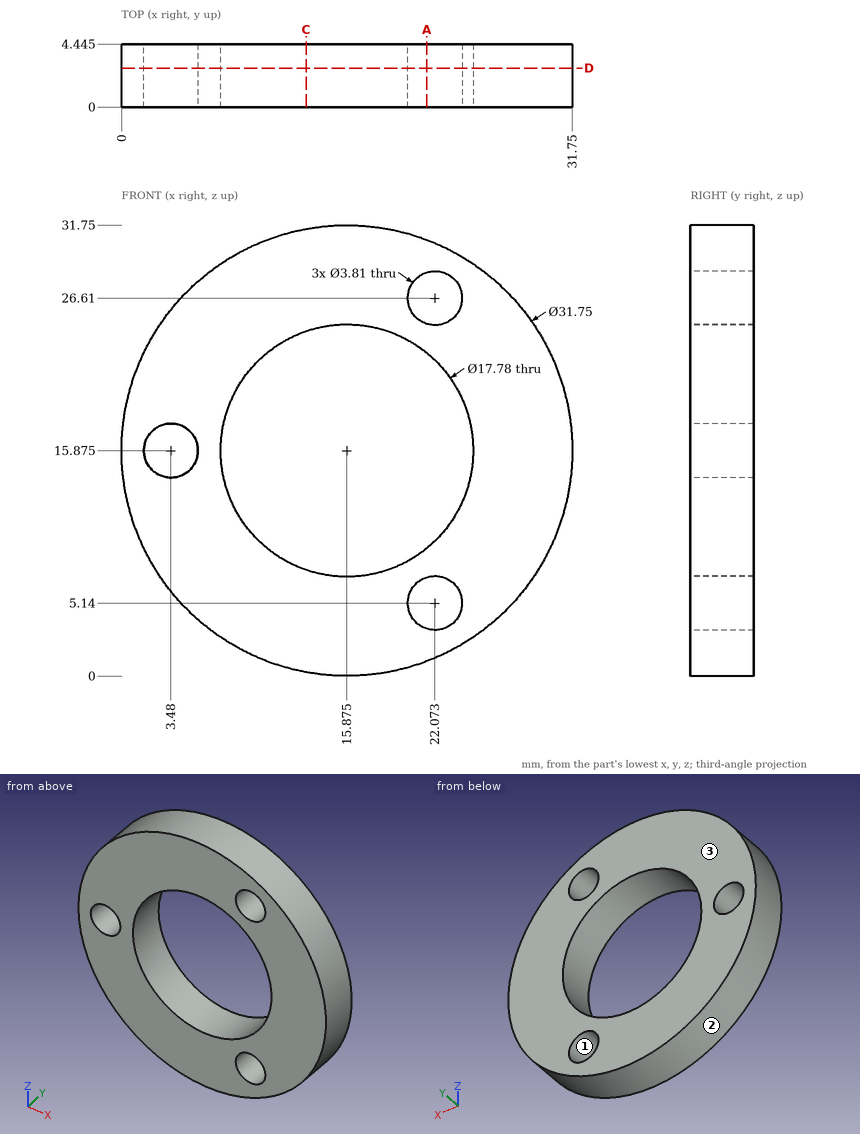
Design review of the part shown in the three views and the two pictorial views. Dimensions are in mm from the part's minimum x, y and z. Give positions to 0.01 mm unless a question says otherwise; leave off trailing zeros. Loops run counter-clockwise (first coordinate to the right, second up) from the corner with the lowest first, then second, coordinate; pieces in that order, holes last. Notation, with made-up numbers: (49.5, 58.5) -> (95.5, 58.5) arc R29 ccw to (95.5, 89.5) -> close; hole circle Ø5 at (34, 18.5). An arc over 180 degrees is marked (long way). Put each result on its own line as item: value. Start each with the question number.
1. Wall thickness on probe 1 along Z at (x, y) = (16, 0.35); probe 2 along X at (y, z) = (0.9, 16.5); probe 3 along X at (y, z) = (0.45, 15.5) (1 decimal): over which ranges is each line inside the solid? List them lowest first.
2. Mouldability with a two-part tool opening along Z and no side actions: class the marked faces 1, 2 and 3 as released by +Z, released by -Z, zero draft, split by the parting line, or undercut.
3. We need section C-C on x = 13. State the section outline as (y, z) points (1 decimal).
4. We need section D-D on y = 2.75. State how many separate pieces and enclosed holes the cut face has, then the cut area to 3 significant figures.
5. Clearance check with flat-ended pins moving along their axes: P1, Ø4.5, axis at x = 22.07, z = 5.14, coming from the -Y side; P2, Ø1, axis at y = 2, z = 17, coming from the +X side; P3, Ø1, axis at y = 1, z = 11.5, coming from the -X side. State where each tip first meets the part, or that it passes through.
6. We need section A-A on x = 21.5. State the section outline as (y, z) points (1 decimal).
Determined:
1. probe 1: 0 to 6.99, 24.76 to 31.75
1. probe 2: 0.01 to 1.68, 5.28 to 7.01, 24.74 to 31.74
1. probe 3: 0 to 1.6, 5.3 to 7, 24.8 to 31.7
2. face 1: undercut
2. face 2: split by the parting line
2. face 3: zero draft
3. outline: (0, 0.3) -> (4.4, 0.3) -> (4.4, 7.5) -> (0, 7.5) -> close; (0, 24.3) -> (4.4, 24.3) -> (4.4, 31.5) -> (0, 31.5) -> close
4. separate pieces: 1
4. enclosed holes: 4
4. area: 509 mm^2
5. P1: y = 0
5. P2: x = 31.74
5. P3: x = 0.48
6. outline: (0, 1) -> (4.4, 1) -> (4.4, 3.3) -> (0, 3.3) -> close; (0, 7) -> (4.4, 7) -> (4.4, 9) -> (0, 9) -> close; (0, 22.8) -> (4.4, 22.8) -> (4.4, 24.8) -> (0, 24.8) -> close; (0, 28.4) -> (4.4, 28.4) -> (4.4, 30.7) -> (0, 30.7) -> close
